Here's how the part is built. I have some questions about the finished solid (model axes, mm). Face numbers are marked on the shaded views. Give positions to 0.01 mm unless a question says otherwise; leave off trailing zeros. Write each loop counter-clockwise with the first axis right and the second up, starting at its lowest first coordinate (ties: lowest second). Pieces come first, ordered by that corner, then holes. Notation, with made-up numbers: (-33.75, 23) - (-3.75, 23) arc R5 ccw to (-3.75, 31) - close; hole circle Ø1 at (12, 11). An arc over 180 degrees is marked (long way). Use one line per item in the form item = value. Start each with the question number.
from build123d import *

# Parameters (mm, degrees)
SKETCH_3_R          = 41
CUT_EXTRUDE_2_DEPTH = 6


with BuildPart() as part:
    # 草图2 → 旋转-薄壁6 (revolve)
    with BuildSketch(Plane.XY, mode=Mode.PRIVATE) as revolve_6_sk:
        Polygon((0, 5.723684211), (50, 5.723684211), (50, -19.276315789), (0, -19.276315789), (0, -17.776315789), (48.5, -17.776315789), (48.5, 4.223684211), (0, 4.223684211), align=None)
    revolve(revolve_6_sk.sketch.rotate(Axis((0, 38.419124221, 0), (0, -1, 0)), 90), axis=Axis((0, 38.419124221, 0), (0, -1, 0)))

    # 草图3 → 切除-拉伸2 (cut, symmetric)
    with BuildSketch(Plane(origin=(0, 0, 0), x_dir=(1, 0, 0), z_dir=(0, 1, 0))):
        with Locations(Location((6.69886917, 0, 0), (0, 0, 270))):
            Circle(SKETCH_3_R)
    extrude(amount=CUT_EXTRUDE_2_DEPTH, both=True, mode=Mode.SUBTRACT)


solid = part.part
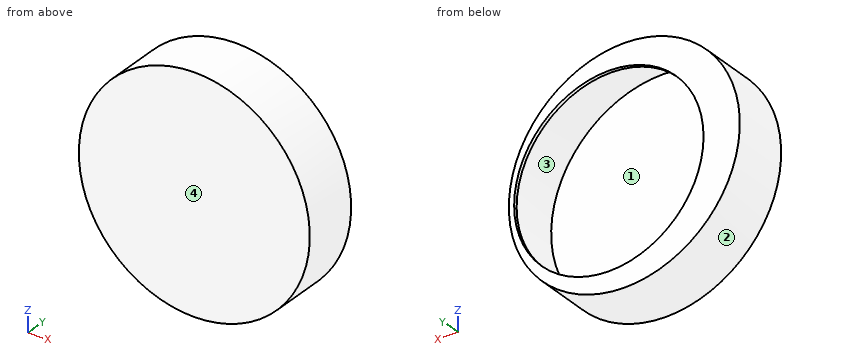
1. We'd pull the mould along Y, two halves only. Please class the marked faces 1, 2, 3 and 4: pulls with the +Y half, pulls with the -Y half, needs draft (parallel to the pull), parting line crosses it, or undercut.
2. For P1, Ø10, axis at x = 16.5, z = -6.5, coming from the +Y side; P2, Ø1, axis at y = -15.5, z = 15, coming from the -X side; P3, Ø8, axis at x = -12.5, y = 1, coming from the -Z side, each with a flat end and sliding along its axis, tell me the tip position at first contact or that it passes through.
3. I want a section at A-A, the plane z = 0. List the corners of the cut face in (x, y) for me.
4. Please list where these lines run through material, in increasing order: line 1 (X direction, y = -1, z = 0); line 2 (Y direction, x = -38, z = -8.5); line 3 (X direction, y = 5.05, z = 0).
5. I want a section at B-B, the plane x = 0. List the corners of the cut face in (y, z) for me, then the cut area to 3 significant figures.
6. I want a section at C-C, the plane y = -15.75. List the corners of the cut face in (x, z) for me, then the cut area to 3 significant figures.
Result sheet:
q1.face_1 = undercut
q1.face_2 = needs draft
q1.face_3 = undercut
q1.face_4 = pulls with the -Y half
q2.P1 = -17.78
q2.P2 = -47.85
q2.P3 = -49.27
q3.outline = (-50, -19.28) - (50, -19.28) - (50, 5.72) - (47.7, 5.72) - (47.7, 4.22) - (48.5, 4.22) - (48.5, -17.78) - (-48.5, -17.78) - (-48.5, 4.22) - (-34.3, 4.22) - (-34.3, 5.72) - (-50, 5.72) - close
q4.line_1 = -50 to -48.5, 48.5 to 50
q4.line_2 = -19.28 to -17.78, 4.22 to 5.72
q4.line_3 = -50 to -34.3, 47.7 to 50
q5.outline = (-19.28, -50) - (5.72, -50) - (5.72, -40.45) - (4.22, -40.45) - (4.22, -48.5) - (-17.78, -48.5) - (-17.78, 48.5) - (4.22, 48.5) - (4.22, 40.45) - (5.72, 40.45) - (5.72, 50) - (-19.28, 50) - close
q5.area = 245 mm2
q6.outline = circle Ø100 at (0, 0); hole circle Ø97 at (0, 0)
q6.area = 464 mm2
